Design review of the part shown in the three views and the two pictorial views. Dimensions are in mm from the part's minimum x, y and z. A direction names the side the tool comes from. Give positions to 0.01 mm unless a question says otherwise; leave off trailing zeros. Order: outer loops, then holes, each group sorted by start corner. A loop starts at its lowest first (then second) coordinate and runs counter-clockwise, first axis right, second up.
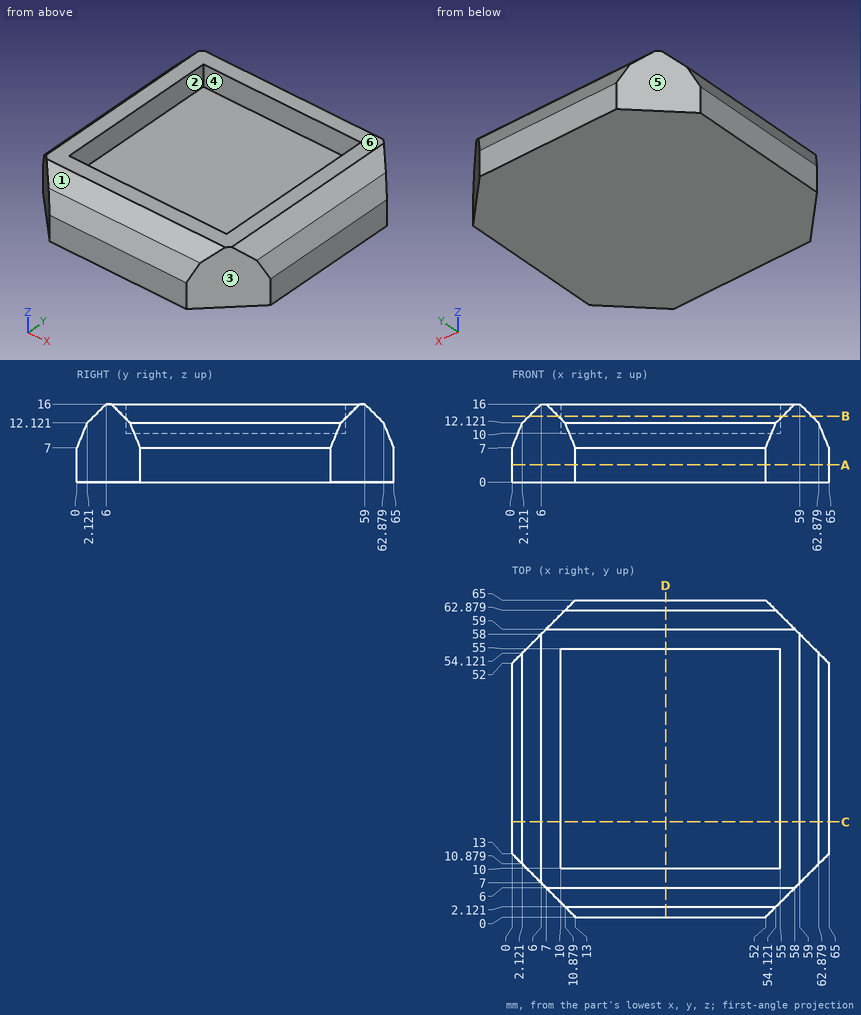
1) We need section B-B on z = 13.5. Give the boundary of the cut face in (x, y).
Answer sheet:
outline: (3.5, 9.5) - (9.5, 3.5) - (55.5, 3.5) - (61.5, 9.5) - (61.5, 55.5) - (55.5, 61.5) - (9.5, 61.5) - (3.5, 55.5) - close; hole (10, 10) - (55, 10) - (55, 55) - (10, 55) - close
2) We need section C-C on y = 19.5. Give the boundary of the cut face in (x, z), then the cut area to 3 significant figures.
Answer sheet:
outline: (0, 0) - (65, 0) - (65, 7) - (62.88, 12.12) - (59, 16) - (55, 16) - (55, 10) - (10, 10) - (10, 16) - (6, 16) - (2.12, 12.12) - (0, 7) - close
area: 728 mm2
3) To check wall thickness, follow line 1 (Z direction, x = 44, y = 11); line 2 (Z direction, x = 24, y = 3); line 3 (Y direction, x = 11.5, z = 15.25). State the ranges of each line that lie inside material, in increasing order.
Answer sheet:
line 1: z = 0 to 10
line 2: z = 0 to 13
line 3: y = 5.25 to 10, 55 to 59.75
4) We need section A-A on z = 3.5. Give the boundary of the cut face in (x, y), then the cut area to 3 significant figures.
Answer sheet:
outline: (0, 13) - (13, 0) - (52, 0) - (65, 13) - (65, 52) - (52, 65) - (13, 65) - (0, 52) - close
area: 3,890 mm2
5) Draft analysis for pull direction X (two halves, no side actions). For the marked faces 3, 4, 5 and 6, state which applies: +X half, -X half, draft (parallel to the pull), parting line (faces both ways), or undercut.
Answer sheet:
face 3: +X half
face 4: undercut
face 5: -X half
face 6: draft
6) Clearance check with flat-ended pins moving along their axes: pin 1 (13.5 mm diameter, centred on x = 36, y = 42.5, fed in from +Z); pin 2 (1 mm diameter, centred on x = 35.5, z = 14, fed in from -Y); pin 3 (1.8 mm diameter, centred on x = 24, z = 13.5, fed in from -Y). State where each tip first meets the part, or that it passes through.
Answer sheet:
pin 1: stops at z = 10
pin 2: stops at y = 3.5
pin 3: stops at y = 2.6
7) Tool access review of the marked faces 1 and 2: name each direction out of +Z, -Z, +X, -X, +Y, -Y from which nothing blocks a thin tool from reaching the whole face with its end or side.
Answer sheet:
face 1: +Z, +X, -X, -Y
face 2: +Z
